Part print with two shaded views. Sizes in mm from the minimum x, y, z corner. Give positions to 0.01 mm unless a question says otherwise; leave off trailing zeros. Write each loop counter-clockwise with the first axis right and the second up, starting at its lowest first coordinate (ties: lowest second). Pieces come first, ordered by that corner, then holes. Notation, with made-up numbers: (78.25, -11.75) -> (113.25, -11.75) arc R12 ccw to (113.25, -6.75) -> close; hole circle Ø6 at (-2, 32). An arc over 180 degrees is marked (long way). Use one line per item in the form item = value. Start each with the question number.
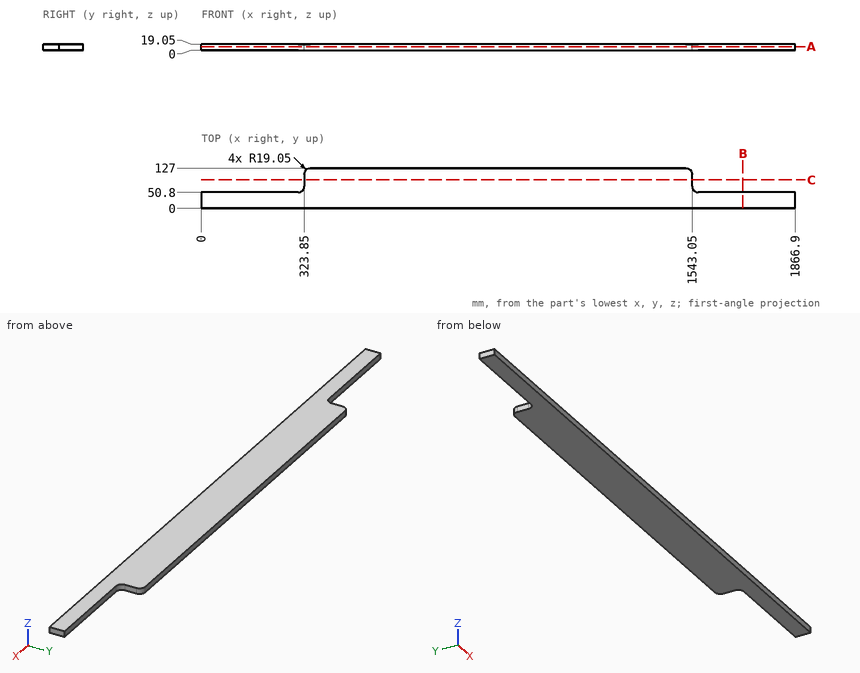
1) Cut at C-C (y = 90). Give the cut face in (x, z).
2) Wall check: line 1 along Y through (x, z) = (1667, 6.5); line 2 along X through (y, z) = (105.5, 13); line 3 along X through (y, z) = (55.5, 2). Give the ranges that are in metal, low to high. Write a range as from..to.
3) Cut at B-B (x = 1703). Give the cut face in (y, z), and give its area (3 significant figures).
4) Cut at A-A (z = 11). Give the cut face in (x, y).
5) Pin check, flat tips, straight feed: pin 1 (1.5 mm diameter, centred on y = 72.5, z = 3.5, fed in from +X); pin 2 (3 mm diameter, centred on y = 97.5, z = 8, fed in from -X); pin 3 (9.5 mm diameter, centred on x = 1642.5, z = 5, fed in from +Y). Stop position of each tip, or through.
Final values:
q1.outline = (323.85, 0) -> (1543.05, 0) -> (1543.05, 19.05) -> (323.85, 19.05) -> close
q2.line_1 = 0..50.8
q2.line_2 = 323.85..1543.05
q2.line_3 = 317.33..1549.57
q3.outline = (0, 0) -> (50.8, 0) -> (50.8, 19.05) -> (0, 19.05) -> close
q3.area = 968 mm^2
q4.outline = (0, 0) -> (1866.9, 0) -> (1866.9, 50.8) -> (1562.1, 50.8) arc R19.05 cw to (1543.05, 69.85) -> (1543.05, 107.95) arc R19.05 ccw to (1524, 127) -> (342.9, 127) arc R19.05 ccw to (323.85, 107.95) -> (323.85, 69.85) arc R19.05 cw to (304.8, 50.8) -> (0, 50.8) -> close
q5.pin_1 = 1543.05
q5.pin_2 = 323.85
q5.pin_3 = 50.8
